Job drawing, mm, ordinate dimensions from the low corner. One solid piece. A direction names the side the tool comes from. Coordinates: 2 decimals unless noted, no trailing zeros. Write each loop counter-clockwise with the first axis right and the second up, starting at its lowest first coordinate (ties: lowest second). Pieces come first, ordered by that corner, then holes. Notation, with made-up numbers: (-10, -25.75) - (25, -25.75) arc R38 cw to (25, 13.25) - close; hole circle Ø6 at (77, 48). An arc over 180 degrees is marked (long way). Use one line per item in the form item = value. Start each with the question number.
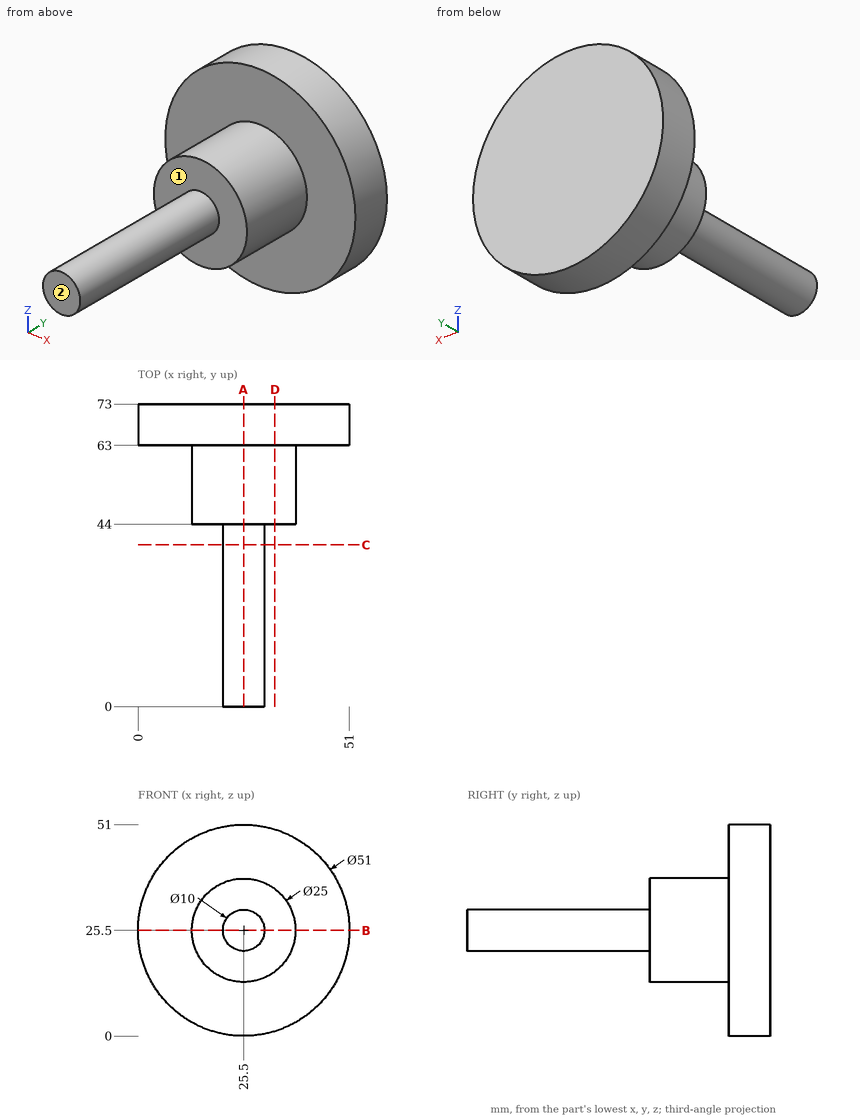
Q1. Drill centre lines: probe 1 along Y at (x, z) = (27.5, 44); probe 2 along X at (y, z) = (54, 25.5); probe 3 along Y at (x, z) = (14.5, 29). Where is each one in solid material? Low to high.
Q2. Slice it at B-B (z = 25.5). List the corners of the cut face in (x, y), plus the area to 4 significant figures.
Q3. Slice it at A-A (x = 25.5). List the corners of the cut face in (y, z).
Q4. Which spindle directions (+Z, -Z, +X, -X, +Y, -Y) get a long thin tool onto all of the face, cutting with end or side? Do the marked faces 1 and 2. Say none if no direction does.
Q5. Slice it at C-C (y = 39). List the corners of the cut face in (x, z), plus the area to 3 significant figures.
Q6. Slice it at D-D (x = 33). List the corners of the cut face in (y, z).
Q7. Pin check, flat tips, straight feed: P1, Ø7.5, axis at x = 30.5, z = 25.5, coming from the -Y side; P2, Ø3, axis at x = 23, y = 21, coming from the -Z side; P3, Ø3, axis at x = 29.5, y = 22.5, coming from the -Z side; P4, Ø5, axis at x = 20.5, y = 59.5, coming from the -Z side. Stop position of each tip, or through.
Solution:
q1.probe_1 = 63 to 73
q1.probe_2 = 13 to 38
q1.probe_3 = 44 to 73
q2.outline = (0, 63) - (13, 63) - (13, 44) - (20.5, 44) - (20.5, 0) - (30.5, 0) - (30.5, 44) - (38, 44) - (38, 63) - (51, 63) - (51, 73) - (0, 73) - close
q2.area = 1,425 mm2
q3.outline = (0, 20.5) - (44, 20.5) - (44, 13) - (63, 13) - (63, 0) - (73, 0) - (73, 51) - (63, 51) - (63, 38) - (44, 38) - (44, 30.5) - (0, 30.5) - close
q4.face_1 = -Y
q4.face_2 = +Z, -Z, +X, -X, -Y
q5.outline = circle Ø10 at (25.5, 25.5)
q5.area = 78.5 mm2
q6.outline = (44, 15.5) - (63, 15.5) - (63, 1.13) - (73, 1.13) - (73, 49.87) - (63, 49.87) - (63, 35.5) - (44, 35.5) - close
q7.P1 = 0
q7.P2 = 20.6
q7.P3 = 21.17
q7.P4 = 13.25
